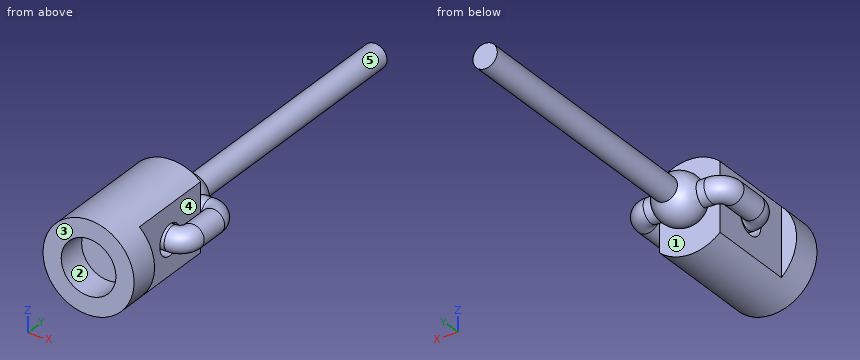
Autodesk Inventor part; units mm, degrees
ref_plane "Work Plane2" through (0, 4.5, 0) normal (0, 1, 0) x (1, 0, 0)
ref_plane "YZ Plane" through (0, 0, 0) normal (1, 0, 0) x (0, 1, 0)
ref_plane "XZ Plane" through (0, 0, 0) normal (0, 1, 0) x (-1, 0, 0)
sketch "스케치2" plane through (0, 0, 0) normal (0, 1, 0) x (-1, 0, 0)
  circle A0 centre (0, 0) radius 1.5
  circle A1 centre (0, 0) radius 0.9
  dimension "d0" = 3
  dimension "d6" = 1.8
extrude "돌출1" add sketch "스케치2" along normal blind 1
sketch "스케치4" plane through (0, 1, 0) normal (0, 1, 0) x (1, 0, 0)
  line L0 (1, -3.1) -> (-1, -3.1)
  line L1 (-1, -3.1) -> (-1, 3.1)
  line L2 (-1, 3.1) -> (1, 3.1)
  line L3 (1, 3.1) -> (1, -3.1)
  line L4 (1, -3.1) -> (-1, 3.1) construction
  line L5 (-1, -3.1) -> (1, 3.1) construction
  circle A0 centre (0, 0) radius 1.5
  point P0 (1, 1.118034)
  point P1 (-1, 1.118034)
  point P2 (-1, -1.118034)
  point P3 (1, -1.118034)
  dimension "d7" = 2
extrude "돌출5" add sketch "스케치4" along normal blind 3 contours A0 L1 L3
sketch "스케치6" plane through (1, 1, 1.118034) normal (1, 0, 0) x (0, 0, -1)
  circle A0 centre (1.118034, 1.5) radius 0.5
  line L0 (0, 3) -> (2.236068, 3)
  point P0 (1.118034, -1)
  dimension "d22" = 1
  dimension "d23" = 1.5
extrude "돌출6" cut sketch "스케치6" along normal through all both and the other way through all
sketch "Sketch7" plane through (0, 4, 0) normal (0, 1, 0) x (1, 0, 0)
  circle A0 centre (0, 0) radius 0.4
  dimension "d26" = 0.8
extrude "Extrusion7" add sketch "Sketch7" along normal blind 10
sketch "Sketch8" plane through (0, 0, 0) normal (0, 0, 1) x (1, 0, 0)
  line L0 (0.264968, 4.4) -> (-1, 4.4)
  line L1 (-1.4, 4) -> (-1.4, 3)
  line L2 (-1, 2.6) -> (0.264968, 2.6)
  line L3 (1, 4) -> (-1, 4)
  line L4 (0.264968, 4.4) -> (1, 4.4)
  line L5 (1.4, 4) -> (1.4, 3)
  line L6 (1, 2.6) -> (0.264968, 2.6)
  line L7 (1, 1) -> (1, 4)
  line L8 (-1, 1) -> (-1, 4)
  arc A0 (-1, 4.4) -> (-1.4, 4) centre (-1, 4) ccw
  arc A1 (1.4, 4) -> (1, 4.4) centre (1, 4) ccw
  line L9 (-1, 3) -> (1, 3)
  arc A2 (-1.4, 3) -> (-1, 2.6) centre (-1, 3) ccw
  arc A3 (1, 2.6) -> (1.4, 3) centre (1, 3) ccw
  point P0 (0, 0)
  dimension "d29" = 0.4
  dimension "d30" = 1.4
  dimension "d32" = 0.4
  dimension "d33" = 0.4
sketch "Sketch9" plane through (0, 0, 0) normal (1, 0, 0) x (0, 1, 0)
  circle A0 centre (4.4, 0) radius 0.39
  line L0 (14, -0.4) -> (14, 0.4)
  line L1 (4, 0.4) -> (4, -0.4)
  point P0 (0, 0)
  dimension "d34" = 0.78
sweep "Sweep1" add profiles "Sketch9" path "Sketch8" path curves L0 A0 L1 A2 L2 L6 A3 L5 A1 L4
ref_plane "Work Plane2" through (0, 4.5, 0) normal (0, 1, 0) x (1, 0, 0)
sketch "Sketch11" plane through (0, 4.5, 0) normal (0, 1, 0) x (1, 0, 0)
  circle A0 centre (0, 0) radius 0.9
  circle A1 centre (0, 0) radius 0.8
  line L0 (0, -0.8) -> (0, 0.8)
  dimension "d40" = 1.6
sketch "Sketch11 outline for Revolution2" plane through (0, 4.5, 0) normal (0, 1, 0) x (1, 0, 0)
  line L0 (0, 0.8) -> (0, -0.8)
  arc A0 (0, -0.8) -> (0, 0.8) centre (0, 0) ccw
revolve "Revolution2" add sketch "Sketch11 outline for Revolution2" angle 360 about axis through (0, 4.5, 0.8) along (0, 0, -1)
properties part number "dummy_anchor_end_3.0mm_w_string"
For this review, take the finished solid that the model builds, in its own axes (mm). Face numbers are marked on the shaded views. A direction names the side the tool comes from. Round coordinates to 2 decimals unless told otherwise and drop trailing zeros. Write each loop counter-clockwise with the first axis right and the second up, starting at its lowest first coordinate (ties: lowest second). Pieces come first, ordered by that corner, then holes. Notation, with made-up numbers: (9.5, 24) - (26.5, 24) arc R7 ccw to (26.5, 28) - close; hole circle Ø2 at (17, -37.5). An arc over 180 degrees is marked (long way). Write item = value, one per line. Start each with the question number.
1. For pin 1 Ø1 at (x, z) = (-0.5, -0.5) entering from +Y; pin 2 Ø1.5 at (y, z) = (1.5, -0.5) entering from +X; pin 3 Ø0.7 at (y, z) = (3, 0.5) entering from +X; pin 4 Ø0.6 at (x, z) = (-1, -0.5) entering from +Y, all flat-tipped, find the tip position at first contact; note any pin that passes through.
2. Consider section A-A on x = 0. State the section outline as (y, z) points.
3. Draft analysis for pull direction Y (two halves, no side actions). For the marked faces 3, 4 and 5, state which applies: released by +Y, released by -Y, zero draft, split by the parting line, or undercut.
4. Consider section D-D on y = 10. State the section outline as (x, z) points.
5. Consider section B-B on z = 0. Give the number of separate pieces and of enclosed holes in the cut face, plus the area to 3 significant figures.
6. For the marked faces 1 and 2, list the 3-axis set-ups (+Z, -Z, +X, -X, +Y, -Y) from which the entire face can be reached by the end or side of a thin tool; tool diameter is ignored.
7. Wall thickness on L1, parallel to Z at x = 0, y = 0.2; L2, parallel to Y at x = 0, z = -1; L3, parallel to Y at x = -0.4, z = 0.6: over which ranges is each line inside the solid? List them lowest first.
Evaluation:
q1.pin_1 = 14
q1.pin_2 = 1.5
q1.pin_3 = 1.76
q1.pin_4 = 4.73
q2.outline = (0, -1.5) - (4, -1.5) - (4, -0.62) arc R0.8 ccw to (5.19, -0.4) - (14, -0.4) - (14, 0.4) - (5.19, 0.4) arc R0.8 ccw to (4, 0.62) - (4, 1.5) - (0, 1.5) - (0, 0.9) - (1, 0.9) - (1, -0.9) - (0, -0.9) - close; circle Ø0.78 at (2.6, 0); hole circle Ø1 at (2.5, 0)
q3.face_3 = released by -Y
q3.face_4 = undercut
q3.face_5 = zero draft
q4.outline = circle Ø0.8 at (0, 0)
q5.separate_pieces = 2
q5.enclosed_holes = 1
q5.area = 19.4 mm2
q6.face_1 = none
q6.face_2 = -Y
q7.L1 = -1.5 to -0.9, 0.9 to 1.5
q7.L2 = 0 to 4
q7.L3 = 1 to 4, 4.15 to 4.85
